Design review of the part built by this model. Coordinates are the model's own, in mm. A direction names the side the tool comes from. Coordinates: 2 decimals unless noted, no trailing zeros. Loops run counter-clockwise (first coordinate to the right, second up) from the corner with the lowest first, then second, coordinate; pieces in that order, holes last. Notation, with made-up numbers: M 51,-8.75 L 101,-8.75 A25 ccw 101,26.25 Z; hole C -32,84.25 d11. An arc over 180 degrees is marked long. Put each result on its own line as item: value. Start each with the question number.
(1) Take a section at A-A, the plane z = 1.95. Give the boundary of the cut face in (x, y), then the cut area to 3 significant figures.
(2) Take a section at D-D, the plane y = 6.35. Give the boundary of the cut face in (x, z) (3 decimals), then the cut area to 3 significant figures.
(3) Clearance check with flat-ended pins moving along their axes: pin 1 (4.5 mm diameter, centred on x = 12.7, y = 6.35, fed in from +Z); pin 2 (1.6 mm diameter, centred on x = -6, z = 2, fed in from -Y). State where each tip first meets the part, or that it passes through.
(4) The part is to be moulded in two halves that separate along X. For faces 4 (the flat face through (13, 39, 0)), 5 (the cylindrical face through (13.223, 29.394, 1.565)), 6 (the cylindrical face through (11.403, 21.085, 1.565)), 7 (the flat face through (-12.7, 51, 2)), say which applies: +X half, -X half, draft (parallel to the pull), parting line (faces both ways), or undercut.
(5) For probe 1 along Y at (x, z) = (12.7, 1.1); probe 2 along X at (y, z) = (32, 1.05); probe 3 along Y at (x, z) = (13, 0.45), list the stretches that pass through material, from the lowest coordinate up. Write a range as [from, to].
(6) Take a section at B-B, the plane x = 31.75. Give the boundary of the cut face in (y, z) (3 decimals), then the cut area to 3 significant figures.
(7) Take a section at C-C, the plane y = 50.8. Give the boundary of the cut face in (x, z) (3 decimals), then the cut area to 4 significant figures.
(8) For faces 1 (the flat face through (13, 0, 2)), 2 (the flat face through (25.4, 19, 2)), 3 (the flat face through (-6, 38.1, 2)), list the 3-axis set-ups (+Z, -Z, +X, -X, +Y, -Y) from which the entire face can be reached by the end or side of a thin tool; tool diameter is ignored.
```python
from build123d import *

# Parameters (mm, degrees)
BOSS_EXTRUDE1_DEPTH = 3.175
SKETCH2_R           = 2.413
CUT_EXTRUDE1_DEPTH  = 75.121121315
SKETCH3_R           = 2.413
CUT_EXTRUDE2_DEPTH  = 75.121121315


with BuildPart() as part:
    # Sketch1 → Boss-Extrude1 (new body)
    with BuildSketch(Plane.XY):
        Polygon((0, 0), (0, 38.1), (-12.7, 38.1), (-12.7, 63.5), (38.1, 63.5), (38.1, 38.1), (25.4, 38.1), (25.4, 0), align=None)
    extrude(amount=BOSS_EXTRUDE1_DEPTH)

    # Sketch2 → Cut-Extrude1 (cut, through all)
    with BuildSketch(Plane(origin=(0, 0, 0), x_dir=(-1, 0, 0), z_dir=(0, 0, -1))):
        with Locations((-19.05, 50.8)):
            Circle(SKETCH2_R)
        with Locations((-6.35, 50.8)):
            Circle(SKETCH2_R)
        with Locations((6.35, 50.8)):
            Circle(SKETCH2_R)
        with Locations((-31.75, 50.8)):
            Circle(SKETCH2_R)
    extrude(amount=-CUT_EXTRUDE1_DEPTH, mode=Mode.SUBTRACT)

    # Sketch3 → Cut-Extrude2 (cut, through all)
    with BuildSketch(Plane(origin=(0, 0, 0), x_dir=(-1, 0, 0), z_dir=(0, 0, -1))):
        with Locations((-12.7, 19.05)):
            Circle(SKETCH3_R)
        with Locations((-12.7, 31.75)):
            Circle(SKETCH3_R)
        with Locations((-12.7, 6.35)):
            Circle(SKETCH3_R)
    extrude(amount=-CUT_EXTRUDE2_DEPTH, mode=Mode.SUBTRACT)


solid = part.part
```
Computed values:
1. outline: M -12.7,38.1 L 0,38.1 L 0,0 L 25.4,0 L 25.4,38.1 L 38.1,38.1 L 38.1,63.5 L -12.7,63.5 Z; hole C -6.35,50.8 d4.83; hole C 6.35,50.8 d4.83; hole C 12.7,6.35 d4.83; hole C 12.7,19.05 d4.83; hole C 12.7,31.75 d4.83; hole C 19.05,50.8 d4.83; hole C 31.75,50.8 d4.83
1. area: 2,130 mm^2
2. outline: M 0,0 L 10.287,0 L 10.287,3.175 L 0,3.175 Z; M 15.113,0 L 25.4,0 L 25.4,3.175 L 15.113,3.175 Z
2. area: 65.3 mm^2
3. pin 1: passes through
3. pin 2: stops at y = 38.1
4. face 4: draft
4. face 5: undercut
4. face 6: undercut
4. face 7: -X half
5. probe 1: y = [0, 3.94], [8.76, 16.64], [21.46, 29.34], [34.16, 63.5]
5. probe 2: x = [0, 10.3], [15.1, 25.4]
5. probe 3: y = [0, 3.96], [8.74, 16.66], [21.44, 29.36], [34.14, 63.5]
6. outline: M 38.1,0 L 48.387,0 L 48.387,3.175 L 38.1,3.175 Z; M 53.213,0 L 63.5,0 L 63.5,3.175 L 53.213,3.175 Z
6. area: 65.3 mm^2
7. outline: M -12.7,0 L -8.763,0 L -8.763,3.175 L -12.7,3.175 Z; M -3.937,0 L 3.937,0 L 3.937,3.175 L -3.937,3.175 Z; M 8.763,0 L 16.637,0 L 16.637,3.175 L 8.763,3.175 Z; M 21.463,0 L 29.337,0 L 29.337,3.175 L 21.463,3.175 Z; M 34.163,0 L 38.1,0 L 38.1,3.175 L 34.163,3.175 Z
7. area: 100.0 mm^2
8. face 1: +Z, -Z, +X, -X, -Y
8. face 2: +Z, -Z, +X, -Y
8. face 3: +Z, -Z, -X, -Y
